Solid Edge part; units mm, degrees
sketch "Sketch1" plane through (0, 0, 0) normal (1, 0, 0) x (0, 1, 0)
  line L0 (3, -3) -> (8, -3)
  line L1 (8, -3) -> (8, 0)
  line L2 (8, 0) -> (11, 0)
  line L3 (11, 0) -> (11, 68)
  line L4 (11, 68) -> (8, 68)
  line L5 (8, 68) -> (8, 71)
  line L6 (8, 71) -> (3, 71)
  line L7 (3, 71) -> (3, 68)
  line L8 (3, 68) -> (0, 68)
  line L9 (0, 68) -> (0, 0)
  line L10 (0, 0) -> (3, 0)
  line L11 (3, 0) -> (3, -3)
  dimension "D1" = 8
  dimension "D2" = 8
  dimension "D3" = 11
  dimension "D4" = 11
extrude "Protrusion1" add sketch "Sketch1" against normal blind 3
properties material "Acier"
Work out the finished part from the listing and answer in its coordinate system (mm). A direction names the side the tool comes from. Give positions to 0.01 mm unless a question says otherwise; leave off trailing zeros. Order: outer loops, then holes, each group sorted by start corner. A loop starts at its lowest first (then second) coordinate and runs counter-clockwise, first axis right, second up. Notation, with made-up numbers: (9, -30.5) - (45, -30.5) arc R33 cw to (45, 5.5) - close; hole circle Ø6 at (61.5, 82.5). An arc over 180 degrees is marked (long way). Answer as CSV lines item,"result". Start each with the question number.
Q1. Find the intervals of material crossed by L1, parallel to Z at x = -1.15, y = 1.5, in increasing order. Write a range as [from, to].
Q2. The part is cut by section A-A (x = -1.3). Write down the section's boundary in (y, z), then the cut area to 3 significant figures.
Q3. The part is cut by section B-B (y = 2). Write down the section's boundary in (x, z).
Q4. For faces 1 (the face through (-1, 2, 68)), 2 (the face through (-1, 3, -1)), 3 (the face through (-1, 9, 0)), 4 (the face through (-1, 8, 69)), determine the directions among +Z, -Z, +X, -X, +Y, -Y from which every point of the face is accessible in a straight line to the end or side of a thin tool.
Q5. Given pin 1 Ø0.9 at (x, y) = (-2, 2) entering from +Z; pin 2 Ø1.5 at (x, z) = (-1.5, -1) entering from -Y; pin 3 Ø1.5 at (x, y) = (-2, 10) entering from -Z; pin 4 Ø1 at (x, z) = (-1, 31.5) entering from -Y, each flat-ended and moving along its own axis, determine where each tip first touches the part or whether it passes through.
Check result:
1,L1,"z = [0, 68]"
2,outline,"(0, 0) - (3, 0) - (3, -3) - (8, -3) - (8, 0) - (11, 0) - (11, 68) - (8, 68) - (8, 71) - (3, 71) - (3, 68) - (0, 68) - close"
2,area,"778 mm²"
3,outline,"(-3, 0) - (0, 0) - (0, 68) - (-3, 68) - close"
4,face 1,"+Z, +X, -X, -Y"
4,face 2,"-Z, +X, -X, -Y"
4,face 3,"-Z, +X, -X, +Y"
4,face 4,"+Z, +X, -X, +Y"
5,pin 1,"stops at z = 68"
5,pin 2,"stops at y = 3"
5,pin 3,"stops at z = 0"
5,pin 4,"stops at y = 0"
